from build123d import *

# Parameters (mm, degrees)
SKETCH_1_W          = 4.8
SKETCH_1_H          = 10
EXTRUDE_1_DEPTH     = 12
CUT_EXTRUDE_1_REACH = 14
SKETCH_4_R          = 1


with BuildPart() as part:
    # Эскиз1 → Бобышка-Вытянуть1 (new body)
    with BuildSketch(Plane.XY):
        Rectangle(SKETCH_1_W, SKETCH_1_H)
    extrude(amount=EXTRUDE_1_DEPTH)

    # Эскиз2 → Отверстие обработанное метчиком M41 (revolve, cut)
    with BuildSketch(Plane(origin=(2.4, 0, 5.5), x_dir=(0, 0, -1), z_dir=(0, 1, 0))):
        Polygon((0, 0), (0, 4.8), (2.275, 4.8), (2, 4.525), (2, 0.275), (2.275, 0), align=None)
    revolve(axis=Axis((8.75, 0, 5.5), (-1, 0, 0)), mode=Mode.SUBTRACT)

    # Эскиз4 → Вырез-Вытянуть1 (cut, up to next)
    with BuildSketch(Plane.XY.offset(12), mode=Mode.PRIVATE) as cut_extrude_1_sk1:
        Circle(SKETCH_4_R)
    cut_extrude_1_tool1 = extrude(cut_extrude_1_sk1.sketch, amount=-CUT_EXTRUDE_1_REACH, mode=Mode.PRIVATE) & part.part
    add(cut_extrude_1_tool1.solids().sort_by_distance((0, 0, 12))[0], mode=Mode.SUBTRACT)


solid = part.part
CAD build for the part. Positions are in the model's coordinates, mm. A direction names the side the tool comes from. Give positions to 0.01 mm unless a question says otherwise; leave off trailing zeros. Order: outer loops, then holes, each group sorted by start corner. A loop starts at its lowest first (then second) coordinate and runs counter-clockwise, first axis right, second up. Notation, with made-up numbers: (-38.5, 14.25) -> (-6.5, 14.25) arc R9 cw to (-6.5, 31.25) -> close; hole circle Ø8 at (-28.75, 38). An arc over 180 degrees is marked (long way). Return JSON: item names as keys, results as strings.
Q1. Flat gauge pin, fed straight in: pin 1 (4.5 mm diameter, centred on y = 0, z = 5.5, fed in from -X) (3 decimals). Where does the tip first touch, or does it go through?
Working result:
{"pin 1": "x = -2.375"}
Q2. Saw through at B-B (y = 0). Write the cut outline in (x, z) (3 decimals), then the cut area to 3 significant figures.
Working result:
{"outline": "(-2.4, 0) -> (2.4, 0) -> (2.4, 3.225) -> (2.125, 3.5) -> (-2.125, 3.5) -> (-2.4, 3.225) -> close; (-2.4, 7.775) -> (-2.125, 7.5) -> (-1, 7.5) -> (-1, 12) -> (-2.4, 12) -> close; (1, 7.5) -> (2.125, 7.5) -> (2.4, 7.775) -> (2.4, 12) -> (1, 12) -> close", "area": "29.2 mm²"}
Q3. Which spindle directions (+Z, -Z, +X, -X, +Y, -Y) get a long thin tool onto all of the face, cutting with end or side? Do faces 1 (the face through (0, -5, 6)), 2 (the face through (0, -1, 10)). Say none if no direction does.
Working result:
{"face 1": "+Z, -Z, +X, -X, -Y", "face 2": "+Z"}
Q4. Drill centre lines: line 1 (Y direction, x = 0, z = 10.05); line 2 (Y direction, x = -1.2, z = 5.5); line 3 (X direction, y = 0, z = 8.2). Where is each one in solid material? Low to high.
Working result:
{"line 1": "-5 to -1, 1 to 5", "line 2": "-5 to -2, 2 to 5", "line 3": "-2.4 to -1, 1 to 2.4"}
Q5. Saw through at A-A (z = 5.5). Write the cut outline in (x, y) (3 decimals), then the cut area to 3 significant figures.
Working result:
{"outline": "(-2.4, -5) -> (2.4, -5) -> (2.4, -2.275) -> (2.125, -2) -> (-2.125, -2) -> (-2.4, -2.275) -> close; (-2.4, 2.275) -> (-2.125, 2) -> (2.125, 2) -> (2.4, 2.275) -> (2.4, 5) -> (-2.4, 5) -> close", "area": "28.6 mm²"}
Q6. Saw through at D-D (x = 1.25). Write the cut outline in (y, z), then the cut area to 3 significant figures.
Working result:
{"outline": "(-5, 0) -> (5, 0) -> (5, 12) -> (-5, 12) -> close; hole circle Ø4 at (0, 5.5)", "area": "107 mm²"}
Q7. Mould opens along Z. For faces 3 (the face through (0.03, 0.766, 3.653)), 4 (the face through (0, 5, 6)), 5 (the face through (0, 1.2, 12)) say: pulls with the +Z half, pulls with the -Z half, needs draft (parallel to the pull), parting line crosses it, or undercut.
Working result:
{"face 3": "undercut", "face 4": "needs draft", "face 5": "pulls with the +Z half"}
Q8. Saw through at C-C (z = 9.75). Write the cut outline in (x, y), then the cut area to 3 significant figures.
Working result:
{"outline": "(-2.4, -5) -> (2.4, -5) -> (2.4, 5) -> (-2.4, 5) -> close; hole circle Ø2 at (0, 0)", "area": "44.9 mm²"}
